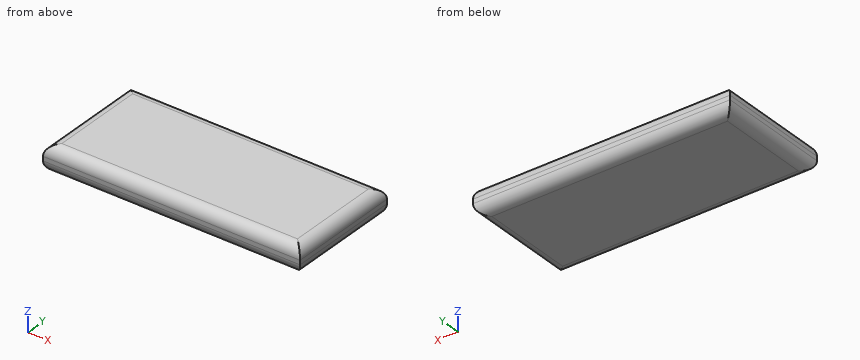
Autodesk Inventor part; units mm, degrees
ref_plane "YZ Plane" through (0, 0, 0) normal (1, 0, 0) x (0, 1, 0)
ref_plane "XZ Plane" through (0, 0, 0) normal (0, 1, 0) x (-1, 0, 0)
ref_plane "XY Plane" through (0, 0, 0) normal (0, 0, 1) x (1, 0, 0)
sketch "Sketch1" plane through (0, 0, 0) normal (0, 0, 1) x (1, 0, 0)
  line L0 (0, 14.98) -> (0, -14.98) construction
  line L1 (-33.6, 0) -> (33.6, 0) construction
  line L2 (24, -10.7) -> (-24, -10.7)
  line L3 (-24, -10.7) -> (-24, 10.7)
  line L4 (-24, 10.7) -> (24, 10.7)
  line L5 (24, 10.7) -> (24, -10.7)
  line L6 (24, -10.7) -> (-24, 10.7) construction
  line L7 (-24, -10.7) -> (24, 10.7) construction
  point P0 (0, 0)
  dimension "d0" = 21.4
  dimension "d1" = 48
extrude "Extrusion1" add sketch "Sketch1" along normal blind 4.8
fillet "Fillet1" radius 2 8 edges at (0, -10.7, 4.8) (0, -10.7, 0) (0, 10.7, 4.8) (0, 10.7, 0) (24, 0, 4.8) (24, 0, 0) (-24, 0, 0) (-24, 0, 4.8)
properties part number "3,.7V 500mAh"
Input: part model. Units: mm. Frame: model coordinates. Give positions to 0.01 mm unless a question says otherwise; leave off trailing zeros. Order: outer loops, then holes, each group sorted by start corner. A loop starts at its lowest first (then second) coordinate and runs counter-clockwise, first axis right, second up.
1. Material intervals for L1, parallel to Y at x = 16, z = 2.9; L2, parallel to X at y = -7, z = 1.05; L3, parallel to Y at x = -4, z = 3.7, sorted ascending.
Derived:
L1: y = -10.7 to 10.7
L2: x = -23.76 to 23.76
L3: y = -10.49 to 10.49
2. Section B-B on z = 0.8. Return the cut outline in (x, y), and give its area (3 significant figures).
Derived:
outline: (-23.6, -10.3) - (23.6, -10.3) - (23.6, 10.3) - (-23.6, 10.3) - close
area: 972 mm2
3. Section A-A on x = -16. Return the cut outline in (y, z).
Derived:
outline: (-10.7, 2) arc R2 ccw to (-8.7, 0) - (8.7, 0) arc R2 ccw to (10.7, 2) - (10.7, 2.8) arc R2 ccw to (8.7, 4.8) - (-8.7, 4.8) arc R2 ccw to (-10.7, 2.8) - close
